Here's the drawing with two shaded views (mm, measured from the low corner). I have some questions. Coordinates: 2 decimals unless noted, no trailing zeros. Write each loop counter-clockwise with the first axis right and the second up, starting at its lowest first coordinate (ties: lowest second). Pieces come first, ordered by that corner, then holes. Notation, with made-up numbers: (42.25, -20) -> (52.25, -20) arc R17 cw to (52.25, 8) -> close; hole circle Ø3 at (8.5, 39). An arc over 180 degrees is marked (long way). Put each result on its own line as item: value.
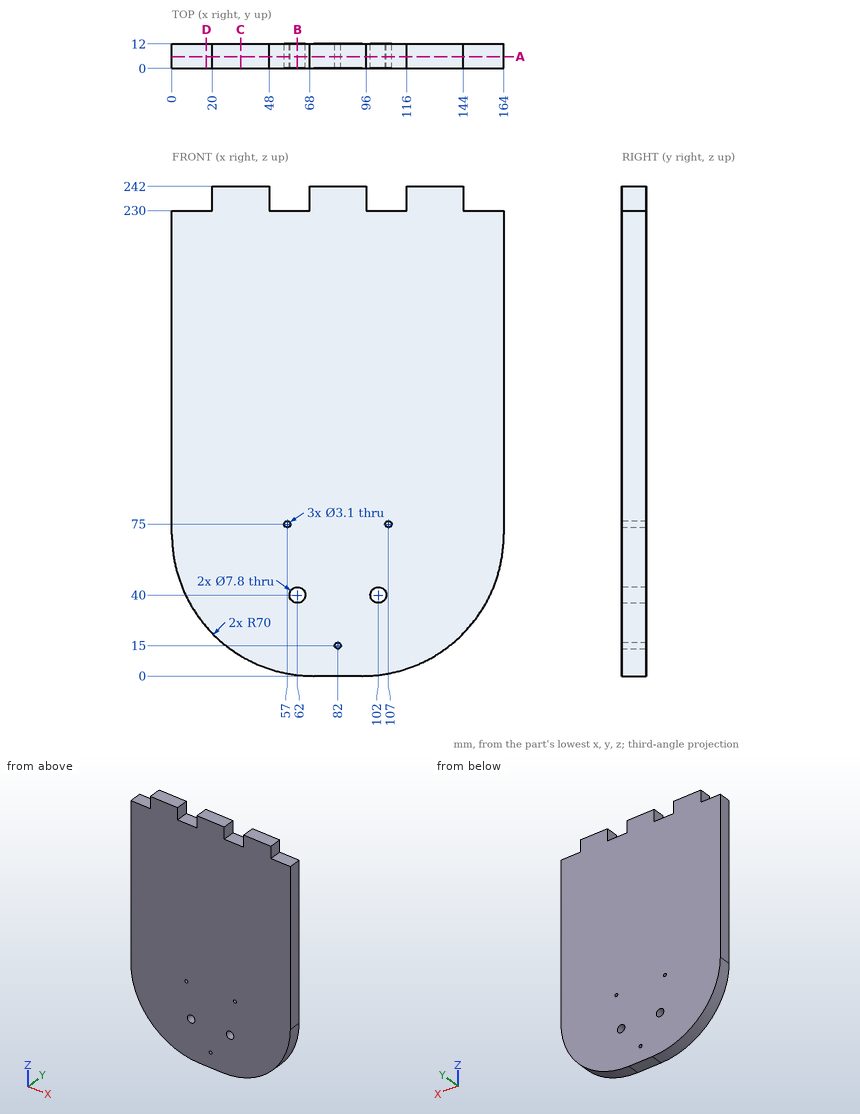
Item 1: Imagine slicing it at A-A on y = 5.75. Write out the boundary of the cut face in (x, z).
Output:
outline: (0, 70) arc R70 ccw to (70, 0) -> (94, 0) arc R70 ccw to (164, 70) -> (164, 230) -> (144, 230) -> (144, 242) -> (116, 242) -> (116, 230) -> (96, 230) -> (96, 242) -> (68, 242) -> (68, 230) -> (48, 230) -> (48, 242) -> (20, 242) -> (20, 230) -> (0, 230) -> close; hole circle Ø3.1 at (57, 75); hole circle Ø7.8 at (62, 40); hole circle Ø3.1 at (82, 15); hole circle Ø7.8 at (102, 40); hole circle Ø3.1 at (107, 75)
Item 2: Please list where these lines run through material, in increasing order: line 1 along X through (y, z) = (9.75, 75); line 2 along X through (y, z) = (3, 40); line 3 along Z through (x, y) = (63.5, 11). Write a range as from..to.
Output:
line 1: x = 0..55.45, 58.55..105.45, 108.55..164
line 2: x = 6.75..58.1, 65.9..98.1, 105.9..157.25
line 3: z = 0.3..36.4, 43.6..230
Item 3: For P1, Ø6, axis at x = 152, y = 9, coming from the +Z side; P2, Ø3.5, axis at y = 6.5, z = 233.5, coming from the -X side; P3, Ø6, axis at y = 6.5, z = 236, coming from the +X side, each with a flat end and sliding along its axis, tell me the tip position at first contact or that it passes through.
Output:
P1: stops at z = 230
P2: stops at x = 20
P3: stops at x = 144
Item 4: Imagine slicing it at C-C on x = 34. Write out the boundary of the cut face in (y, z), then the cut area to 3 significant figures.
Output:
outline: (0, 9.97) -> (12, 9.97) -> (12, 242) -> (0, 242) -> close
area: 2,780 mm²
Item 5: Imagine slicing it at D-D on x = 17. Write out the boundary of the cut face in (y, z), then the cut area to 3 significant figures.
Output:
outline: (0, 24.27) -> (12, 24.27) -> (12, 230) -> (0, 230) -> close
area: 2,470 mm²
Item 6: Imagine slicing it at B-B on x = 62. Write out the boundary of the cut face in (y, z).
Output:
outline: (0, 0.46) -> (12, 0.46) -> (12, 36.1) -> (0, 36.1) -> close; (0, 43.9) -> (12, 43.9) -> (12, 230) -> (0, 230) -> close
